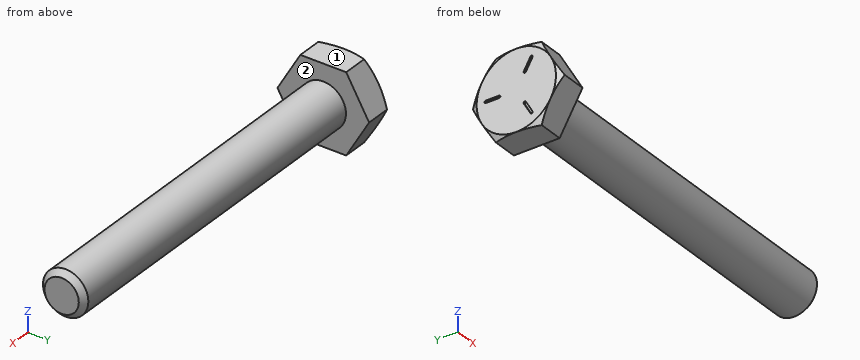
from build123d import *

# Parameters (mm, degrees)
SKETCH5_R           = 3.175
BOSS_EXTRUDE3_DEPTH = 50.8
CHAMFER1_SIZE       = 0.77724
BOSS_EXTRUDE4_DEPTH = 3.96875
SKETCH8_OUTSIDE_W   = 217.768
SKETCH8_OUTSIDE_H   = 219.488
SKETCH8_OUTSIDE_R   = 5.55625
CUT_EXTRUDE3_DEPTH  = 55.76875
CUT_EXTRUDE3_TAPER  = 60
CUT_EXTRUDE4_DEPTH  = 0.254
CIRPATTERN1_COUNT   = 3


with BuildPart() as part:
    # Sketch5 → Boss-Extrude3 (new body)
    with BuildSketch(Plane(origin=(27.384375, 0, 0), x_dir=(0, 0, -1), z_dir=(1, 0, 0))):
        Circle(SKETCH5_R)
    extrude(amount=-BOSS_EXTRUDE3_DEPTH)

    # Chamfer1
    chamfer1_edges = [part.edges().sort_by_distance(p)[0] for p in [
        (27.384375, 0, 3.175),
    ]]
    chamfer(chamfer1_edges, length=CHAMFER1_SIZE)

    # Sketch6 → Boss-Extrude4 (add)
    with BuildSketch(Plane.ZY.offset(23.415625)):
        Polygon((5.55625, 3.207902433), (0, 6.415804866), (-5.55625, 3.207902433), (-5.55625, -3.207902433), (0, -6.415804866), (5.55625, -3.207902433), align=None)
    extrude(amount=BOSS_EXTRUDE4_DEPTH)

    # Sketch8 outside → Cut-Extrude3 (cut, through all)
    with BuildSketch(Plane.ZY.offset(27.384375)):
        Rectangle(SKETCH8_OUTSIDE_W, SKETCH8_OUTSIDE_H)
        Circle(SKETCH8_OUTSIDE_R, mode=Mode.SUBTRACT)
    extrude(amount=-CUT_EXTRUDE3_DEPTH, taper=CUT_EXTRUDE3_TAPER, mode=Mode.SUBTRACT)

    # Sketch12 → Cut-Extrude4 (cut)
    with BuildSketch(Plane.ZY.offset(27.384375)):
        with BuildLine():
            Line((0.1666875, 4.2783125), (0.1666875, 2.3891875))
            ThreePointArc((0.1666875, 2.3891875), (0, 2.2225), (-0.1666875, 2.3891875))
            Line((-0.1666875, 2.3891875), (-0.1666875, 4.2783125))
            ThreePointArc((-0.1666875, 4.2783125), (0, 4.445), (0.1666875, 4.2783125))
        make_face()
    cut_extrude4 = extrude(amount=-CUT_EXTRUDE4_DEPTH, mode=Mode.SUBTRACT)

    # CirPattern1: Cut-Extrude4 ×3 about axis
    cirpattern1_axis = Axis((0, 0, 0), (1, 0, 0))
    for i in range(1, CIRPATTERN1_COUNT):
        add(cut_extrude4.rotate(cirpattern1_axis, i * 360 / CIRPATTERN1_COUNT), mode=Mode.SUBTRACT)


solid = part.part
Input: part model. Units: mm. Frame: model coordinates. Face numbers are marked on the shaded views. A direction names the side the tool comes from. Coordinates: 2 decimals unless noted, no trailing zeros. Order: outer loops, then holes, each group sorted by start corner. A loop starts at its lowest first (then second) coordinate and runs counter-clockwise, first axis right, second up. Notation, with made-up numbers: M 4,61 L 12,61 A33 ccw 12,91 Z; hole C 40,26 d2. An arc over 180 degrees is marked long. One line per question, with ' | ' between items.
Item 1: Pin query (flat end, axial travel): pin 1 (5 mm diameter, centred on x = 0, y = -4.5, fed in from +Z); pin 2 (3 mm diameter, centred on x = -11, y = -3, fed in from +Z); pin 3 (1 mm diameter, centred on y = -1.5, z = 2.5, fed in from -X); pin 4 (3 mm diameter, centred on x = 9.5, y = 2, fed in from +Z). Return the tip coordinate at first contact, or that it passes through.
Geometry results:
pin 1: stops at z = 2.47 | pin 2: stops at z = 2.8 | pin 3: stops at x = -27.38 | pin 4: stops at z = 3.14
Item 2: Ray query, line 1 along Y through (x, z) = (-5.5, 0) (3 decimals); line 2 along X through (y, z) = (-4.25, -2.5); line 3 along X through (y, z) = (2, -1.5). Return the intervals inside material, ascending.
Geometry results:
line 1: y = -3.175 to 3.175 | line 2: x = -27.38 to -23.42 | line 3: x = -27.38 to 27.28
Item 3: Section A-A (x = -13.5). Output: boundary loops of the cut face in (y, z) (3 decimals).
Geometry results:
outline: C 0,0 d6.35
Item 4: Reachability of the marked faces 1 and 2 from +Z, -Z, +X, -X, +Y, -Y: full face, straight path, thin tool, end or side. Return the list, or none.
Geometry results:
face 1: +Z, +X, -X, +Y, -Y | face 2: +X
